Input: part model. Units: mm. Frame: model coordinates. A direction names the side the tool comes from. Give positions to 0.01 mm unless a question says otherwise; leave off trailing zeros. Write each loop counter-clockwise with the first axis right and the second up, starting at its lowest first coordinate (ties: lowest second). Pieces come first, ordered by that corner, then holes. Notation, with made-up numbers: (31.25, 77.25) - (72.25, 77.25) arc R30 cw to (72.25, 109.25) - close; hole circle Ø6 at (-1, 60.25). An arc over 180 degrees is marked (long way). Use a Markdown table: item, result. Add a question column.
1. Pin query (flat end, axial travel): pin 1 (4 mm diameter, centred on y = 5.5, z = 9, fed in from +X); pin 2 (0.6 mm diameter, centred on x = 5.5, z = -1, fed in from -Y); pin 3 (5 mm diameter, centred on x = 8, z = 5, fed in from +Y). Return the tip coordinate at first contact, or that it passes through.
2. Section query C-C, the plane z = 9. Return loops of the section in (x, y), plus the area to 3 significant figures.
3. Section query D-D, the plane y = 1.5. Return loops of the section in (x, z), plus the area to 3 significant figures.
4. Material intervals for probe 1 along Z at (x, y) = (1.5, 4.5); probe 2 along Y at (x, z) = (11.7, 1.2); probe 3 along Y at (x, z) = (4.2, 7.6), sorted ascending.
5. Set-up query: faces 1 (the cylindrical face through (0.4, 12.5, 2.3)), 2 (the flat face through (10, 5.6, 1)), 3 (the flat face through (4, 6, 0)). Return all of +Z, -Z, +X, -X, +Y, -Y with unobstructed straight access to the full face (end or side cutting, diameter ignored); none if empty.
6. Mould query, pull axis Y, two halves, no side actions, for faces 4 (the flat face through (1.123, 12.008, 5.639)), 5 (the cylindrical face through (13.9, 6.02, 0.89)), 6 (the flat face through (4, 11.4, 3)). Classes: released by +Y, released by -Y, zero draft, split by the parting line, or undercut.
7. Section query B-B, the plane y = 10.3. Return loops of the section in (x, z).
```python
from build123d import *

# Parameters (mm, degrees)
EXTRUDE_1_DEPTH      = 10.8
SKETCH_2_R           = 1
EXTRUDE_2_DEPTH      = 0.8
SKETCH_3_W           = 1.7
SKETCH_3_H           = 8.1
CUT_EXTRUDE_1_DEPTH  = 17.8
EXTRUDE_START        = -4.5
EXTRUDE_3_DEPTH      = 4.5
SKETCH_5_W           = 8.4
SKETCH_5_H           = 0.05
CUT_EXTRUDE_2_DEPTH  = 1
SKETCH_6_R           = 1
CUT_EXTRUDE_3_DEPTH  = 8
CUT_EXTRUDE_4_DEPTH  = 1.2
SKETCH_8_W           = 2.8
SKETCH_8_H           = 0.608363533
EXTRUDE_4_DEPTH      = 0.1
EXTRUDE_START_2      = 2.5
EXTRUDE_5_DEPTH      = 2.5
SKETCH_10_W          = 8.4
SKETCH_10_H          = 1.7
CUT_EXTRUDE_5_DEPTH  = 0.05
FILLET_1_R           = 1.4
SKETCH_11_W          = 0.05
SKETCH_11_H          = 5.83834946
SKETCH_11_H_2        = 5.828769054
CUT_EXTRUDE_8_DEPTH  = 0.05
SKETCH_12_R          = 1.4
CUT_EXTRUDE_9_DEPTH  = 4
SKETCH_13_W          = 0.5
SKETCH_13_H          = 5.54
EXTRUDE_6_DEPTH      = 1.45
FILLET_2_R           = 1
CUT_EXTRUDE_START    = -8.12
CUT_EXTRUDE_10_DEPTH = 8.12


with BuildPart() as part:
    # Эскиз1 → Бобышка-Вытянуть1 (new body)
    with BuildSketch(Plane.XY):
        Polygon((7.4, 0), (8.4, 1), (8.4, 12.6), (0, 12.6), (0, 1), (1, 0), align=None)
    extrude(amount=EXTRUDE_1_DEPTH)

    # Эскиз2 → Бобышка-Вытянуть2 (add)
    with BuildSketch(Plane(origin=(0, 0, 0), x_dir=(-1, 0, 0), z_dir=(0, 0, -1))):
        with Locations((-4.2, 10.3)):
            Circle(SKETCH_2_R)
        with Locations((-4.2, 3.9)):
            Circle(SKETCH_2_R)
    extrude(amount=EXTRUDE_2_DEPTH)

    # Эскиз3 → Вырез-Вытянуть1 (cut)
    with BuildSketch(Plane(origin=(8.4, 0, 0), x_dir=(0, 0, -1), z_dir=(1, 0, 0))):
        with Locations((-4.75, 4.05)):
            Rectangle(SKETCH_3_W, SKETCH_3_H)
    extrude(amount=-CUT_EXTRUDE_1_DEPTH, mode=Mode.SUBTRACT)

    # Эскиз4 → Бобышка-Вытянуть3 (add)
    with BuildSketch(Plane(origin=(0, 12.6, 0), x_dir=(1, 0, 0), z_dir=(0, 1, 0)).offset(EXTRUDE_START)):
        with BuildLine():
            Line((9.1, -10.8), (-0.7, -10.8))
            Line((-0.7, -10.8), (-0.7, -2.8))
            ThreePointArc((-0.7, -2.8), (-0.992893219, -2.092893219), (-1.7, -1.8))
            Line((-1.7, -1.8), (-5.9, -1.8))
            Line((-5.9, -1.8), (-5.9, 0))
            Line((-5.9, 0), (14.3, 0))
            Line((14.3, 0), (14.3, -1.8))
            Line((14.3, -1.8), (10.1, -1.8))
            ThreePointArc((10.1, -1.8), (9.392893219, -2.092893219), (9.1, -2.8))
            Line((9.1, -2.8), (9.1, -10.8))
        make_face()
    extrude(amount=EXTRUDE_3_DEPTH)

    # Эскиз5 → Вырез-Вытянуть2 (cut)
    with BuildSketch(Plane.XY.offset(10.8)):
        with Locations((4.2, 8.075)):
            Rectangle(SKETCH_5_W, SKETCH_5_H)
    extrude(amount=-CUT_EXTRUDE_2_DEPTH, mode=Mode.SUBTRACT)

    # Эскиз6 → Вырез-Вытянуть3 (cut)
    with BuildSketch(Plane.XY.offset(10.8)):
        with Locations((4.2, 4)):
            Circle(SKETCH_6_R)
    extrude(amount=-CUT_EXTRUDE_3_DEPTH, mode=Mode.SUBTRACT)

    # Эскиз7 → Вырез-Вытянуть4 (cut)
    with BuildSketch(Plane(origin=(0, 12.6, 0), x_dir=(1, 0, 0), z_dir=(0, 1, 0))):
        with BuildLine():
            Line((8.6, 0), (8.6, -7.112411136))
            ThreePointArc((8.6, -7.112411136), (8.468198052, -7.430609188), (8.15, -7.562411136))
            Line((8.15, -7.562411136), (7.983405928, -7.562411136))
            ThreePointArc((7.983405928, -7.562411136), (7.691564003, -7.454943311), (7.539115931, -7.183870205))
            Line((7.539115931, -7.183870205), (7.049736844, -4.141202068))
            ThreePointArc((7.049736844, -4.141202068), (6.710963351, -3.53881739), (6.062425739, -3.3))
            Line((6.062425739, -3.3), (2.361664993, -3.3))
            ThreePointArc((2.361664993, -3.3), (1.71573807, -3.536600753), (1.37546474, -4.13444318))
            Line((1.37546474, -4.13444318), (0.863036378, -7.186911705))
            ThreePointArc((0.863036378, -7.186911705), (0.709913379, -7.455940797), (0.419246264, -7.562411136))
            Line((0.419246264, -7.562411136), (0.25, -7.562411136))
            ThreePointArc((0.25, -7.562411136), (-0.068198052, -7.430609188), (-0.2, -7.112411136))
            Line((-0.2, -7.112411136), (-0.2, 0))
            Line((-0.2, 0), (8.6, 0))
        make_face()
        with BuildLine():
            Line((4.2, -10.8), (5.6, -10.8))
            Line((5.6, -10.8), (5.6, -5.056380156))
            ThreePointArc((5.6, -5.056380156), (5.453553391, -4.702826765), (5.1, -4.556380156))
            Line((5.1, -4.556380156), (3.3, -4.556380156))
            ThreePointArc((3.3, -4.556380156), (2.946446609, -4.702826765), (2.8, -5.056380156))
            Line((2.8, -5.056380156), (2.8, -10.8))
            Line((2.8, -10.8), (4.2, -10.8))
        make_face()
    extrude(amount=-CUT_EXTRUDE_4_DEPTH, mode=Mode.SUBTRACT)

    # Эскиз8 → Бобышка-Вытянуть4 (add)
    with BuildSketch(Plane(origin=(0, 11.4, 0), x_dir=(1, 0, 0), z_dir=(0, 1, 0))):
        with Locations((4.2, -10.495818233)):
            Rectangle(SKETCH_8_W, SKETCH_8_H)
    extrude(amount=EXTRUDE_4_DEPTH)

    # Эскиз9 → Бобышка-Вытянуть5 (add)
    with BuildSketch(Plane.XZ.offset(-8.1).offset(EXTRUDE_START_2)):
        with BuildLine():
            Line((0, 0), (0, 3.7))
            Line((0, 3.7), (-0.7, 3.7))
            Line((-0.7, 3.7), (-0.7, 2.8))
            ThreePointArc((-0.7, 2.8), (-0.992893219, 2.092893219), (-1.7, 1.8))
            Line((-1.7, 1.8), (-5.9, 1.8))
            Line((-5.9, 1.8), (-5.9, 0))
            Line((-5.9, 0), (0, 0))
        make_face()
        with BuildLine():
            Line((14.3, 0), (8.4, 0))
            Line((8.4, 0), (8.4, 3.7))
            Line((8.4, 3.7), (9.1, 3.7))
            Line((9.1, 3.7), (9.1, 2.8))
            ThreePointArc((9.1, 2.8), (9.392893219, 2.092893219), (10.1, 1.8))
            Line((10.1, 1.8), (14.3, 1.8))
            Line((14.3, 1.8), (14.3, 0))
        make_face()
    extrude(amount=-EXTRUDE_5_DEPTH)

    # Эскиз10 → Вырез-Вытянуть5 (cut)
    with BuildSketch(Plane.XZ.offset(-8.1)):
        with Locations((4.2, 4.75)):
            Rectangle(SKETCH_10_W, SKETCH_10_H)
    extrude(amount=-CUT_EXTRUDE_5_DEPTH, mode=Mode.SUBTRACT)

    # Скругление1
    fillet_1_edges = [part.edges().sort_by_distance(p)[0] for p in [
        (-5.9, 5.6, 0.9),
        (14.3, 5.6, 0.9),
        (14.3, 12.6, 0.9),
        (-5.9, 12.6, 0.9),
    ]]
    fillet(fillet_1_edges, radius=FILLET_1_R)

    # Эскиз11 → Вырез-Вытянуть8 (cut)
    with BuildSketch(Plane(origin=(0, 0, 0), x_dir=(-1, 0, 0), z_dir=(0, 0, -1))):
        with Locations((-8.375, 8.48082527)):
            Rectangle(SKETCH_11_W, SKETCH_11_H)
        with Locations((-0.025, 8.485615473)):
            Rectangle(SKETCH_11_W, SKETCH_11_H_2)
    extrude(amount=-CUT_EXTRUDE_8_DEPTH, mode=Mode.SUBTRACT)

    # Эскиз12 → Вырез-Вытянуть9 (cut)
    with BuildSketch(Plane(origin=(0, 0, 0), x_dir=(-1, 0, 0), z_dir=(0, 0, -1))):
        with Locations((-11.7, 8.24)):
            Circle(SKETCH_12_R)
        with Locations((3.3, 8.24)):
            Circle(SKETCH_12_R)
    extrude(amount=-CUT_EXTRUDE_9_DEPTH, mode=Mode.SUBTRACT)

    # Эскиз13 → Бобышка-Вытянуть6 (add)
    with BuildSketch(Plane(origin=(0, 11.4, 0), x_dir=(1, 0, 0), z_dir=(0, 1, 0))):
        with Locations((5.47, 0.23)):
            Rectangle(SKETCH_13_W, SKETCH_13_H)
        with Locations((8.01, 0.23)):
            Rectangle(SKETCH_13_W, SKETCH_13_H)
        with Locations((2.93, 0.23)):
            Rectangle(SKETCH_13_W, SKETCH_13_H)
        with Locations((0.39, 0.23)):
            Rectangle(SKETCH_13_W, SKETCH_13_H)
    extrude(amount=EXTRUDE_6_DEPTH)

    # Скругление2
    fillet_2_edges = [part.edges().sort_by_distance(p)[0] for p in [
        (5.47, 12.85, 2.54),
        (2.93, 12.85, 2.54),
        (0.39, 12.85, 2.54),
        (8.01, 12.85, 2.54),
    ]]
    fillet(fillet_2_edges, radius=FILLET_2_R)

    # Эскиз14 → Вырез-Вытянуть10 (cut)
    with BuildSketch(Plane.ZY.offset(-0.14).offset(CUT_EXTRUDE_START)):
        with BuildLine():
            Line((-3, 12.6), (1.54, 12.6))
            ThreePointArc((1.54, 12.6), (2.070330086, 12.380330086), (2.29, 11.85))
            Line((2.29, 11.85), (2.29, 11.4))
            Line((2.29, 11.4), (-3, 11.4))
            Line((-3, 11.4), (-3, 12.6))
        make_face()
    extrude(amount=CUT_EXTRUDE_10_DEPTH, mode=Mode.SUBTRACT)


solid = part.part
```
Result sheet:
| question | item | result |
|---|---|---|
| 1 | pin 1 | stops at x = 8.4 |
| 1 | pin 2 | stops at y = 12.6 |
| 1 | pin 3 | stops at y = 12.6 |
| 2 | outline | (-0.7, 8.1) - (0, 8.1) - (0, 1) - (1, 0) - (7.4, 0) - (8.4, 1) - (8.4, 8.1) - (9.1, 8.1) - (9.1, 12.6) - (5.6, 12.6) - (5.6, 11.4) - (2.8, 11.4) - (2.8, 12.6) - (-0.7, 12.6) - close; hole circle Ø2 at (4.2, 4) |
| 2 | area | 105 mm² |
| 3 | outline | (0, 0) - (8.4, 0) - (8.4, 3.9) - (0, 3.9) - close; (0, 5.6) - (8.4, 5.6) - (8.4, 10.8) - (0, 10.8) - close |
| 3 | area | 76.4 mm² |
| 4 | probe 1 | z = 0 to 3.9, 5.6 to 10.8 |
| 4 | probe 2 | y = 5.6 to 6.84, 9.64 to 12.6 |
| 4 | probe 3 | y = 0 to 3, 5 to 11.4 |
| 5 | face 1 | +Y |
| 5 | face 2 | +Z, -Z, +X, -Y |
| 5 | face 3 | -Z |
| 6 | face 4 | zero draft |
| 6 | face 5 | released by -Y |
| 6 | face 6 | undercut |
| 7 | outline | (-5.9, 0) - (0, 0) - (0, 0.05) - (0.05, 0.05) - (0.05, 0) - (3.2, 0) - (3.2, -0.8) - (5.2, -0.8) - (5.2, 0) - (8.35, 0) - (8.35, 0.05) - (8.4, 0.05) - (8.4, 0) - (14.3, 0) - (14.3, 1.8) - (10.1, 1.8) arc R1 cw to (9.1, 2.8) - (9.1, 10.8) - (-0.7, 10.8) - (-0.7, 2.8) arc R1 cw to (-1.7, 1.8) - (-5.9, 1.8) - close |
